from build123d import *

# Parameters (mm, degrees)
F0_W     = 75
F0_H     = 58
F1_DEPTH = 10.5
F3_R     = 5.24999
F4_DEPTH = 6
F5_W     = 6.9
F5_H     = 0.25
F6_DEPTH = 4.572


# Not quite as in the source:
# - a fillet or chamfer is up to 0.001 mm smaller than in the source, because OpenCascade refuses the exact size


with BuildPart() as f1:
    # F0 (on Top) → F1 (new body)
    with BuildSketch(Plane.XY):
        with Locations((-17.9516240954, -13.4977242947)):
            Rectangle(F0_W, F0_H)
    extrude(amount=F1_DEPTH)

    # F3 (radius 5.25 in the source; OpenCascade refuses exactly that, so slightly less here)
    f3_edges = [f1.edges().sort_by_distance(p)[0] for p in [
        (-17.951624, -42.497724, 10.5),
        (-17.951624, -42.497724, 0),
        (-17.951624, 15.502276, 10.5),
        (-17.951624, 15.502276, 0),
    ]]
    fillet(f3_edges, radius=F3_R)

    # F2 (on face) → F4 (cut)
    with BuildSketch(Plane.YZ.offset(19.5483759046)):
        with BuildLine():
            Line((-10.0477242947, 8), (-13.4977242947, 8))
            Line((-13.4977242947, 8), (-16.9477242947, 8))
            ThreePointArc((-16.9477242947, 8), (-15.8517087838, 7.5460155108), (-15.3977242947, 6.45))
            ThreePointArc((-15.3977242947, 6.45), (-15.8517087838, 5.3539844892), (-16.9477242947, 4.9))
            Line((-16.9477242947, 4.9), (-10.0477242947, 4.9))
            ThreePointArc((-10.0477242947, 4.9), (-11.5977242947, 6.45), (-10.0477242947, 8))
        make_face()
        with BuildLine():
            Line((-10.0477242947, 4.9), (-10.0477242947, 8))
            ThreePointArc((-10.0477242947, 8), (-11.5977242947, 6.45), (-10.0477242947, 4.9))
        make_face()
        with BuildLine():
            ThreePointArc((-8.4977242947, 6.45), (-8.9517087838, 7.5460155108), (-10.0477242947, 8))
            Line((-10.0477242947, 8), (-10.0477242947, 4.9))
            ThreePointArc((-10.0477242947, 4.9), (-8.9517087838, 5.3539844892), (-8.4977242947, 6.45))
        make_face()
        with BuildLine():
            ThreePointArc((-15.3977242947, 6.45), (-15.8517087838, 7.5460155108), (-16.9477242947, 8))
            Line((-16.9477242947, 8), (-16.9477242947, 4.9))
            ThreePointArc((-16.9477242947, 4.9), (-15.8517087838, 5.3539844892), (-15.3977242947, 6.45))
        make_face()
        with BuildLine():
            Line((-16.9477242947, 4.9), (-16.9477242947, 8))
            ThreePointArc((-16.9477242947, 8), (-18.0437398055, 7.5460155108), (-18.4977242947, 6.45))
            ThreePointArc((-18.4977242947, 6.45), (-18.0437398055, 5.3539844892), (-16.9477242947, 4.9))
        make_face()
    extrude(amount=-F4_DEPTH, mode=Mode.SUBTRACT)

    # F5 (on face) → F6 (join)
    with BuildSketch(Plane.YZ.offset(13.5483759046)):
        with Locations((-13.4977242947, 6.575)):
            Rectangle(F5_W, F5_H)
        with Locations((-13.4977242947, 6.325)):
            Rectangle(F5_W, F5_H)
    extrude(amount=F6_DEPTH)


solid = f1.part
Check sheet for the modelled part. Datum: model origin and axes. Units: mm. A direction names the side the tool comes from. Round coordinates to 2 decimals unless told otherwise and drop trailing zeros. Loops run counter-clockwise (first coordinate to the right, second up) from the corner with the lowest first, then second, coordinate; pieces in that order, holes last. Notation, with made-up numbers: (35.5, 37.5) -> (58.5, 37.5) arc R34 cw to (58.5, 68.5) -> close; hole circle Ø6 at (25.5, 5). An arc over 180 degrees is marked (long way). Put each result on its own line as item: value. Start each with the question number.
1. Gauge pin test, flat ends, axial feed: pin 1 (5 mm diameter, centred on x = -46.5, z = 1.5, fed in from -Y); pin 2 (0.6 mm diameter, centred on y = -13.5, z = 6.5, fed in from +X); pin 3 (3 mm diameter, centred on x = -17, z = 3.5, fed in from -Y). Record the tip position at first contact, or that the pin passes through.
2. Section check C-C (z = 1.25). Enter the section's corners in (x, y).
3. Draft check along Z on faces 3 (the face through (-17.427, 14.005, 8.921)), 4 (the face through (13.548, -14, 6)), 5 (the face through (-18, -13, 0)). Enter one of: +Z half, -Z half, draft (parallel to the pull), parting line (faces both ways), or undercut.
4. Scan lines: probe 1 along X at (y, z) = (-17.5, 5.5); probe 2 along Z at (x, y) = (-26, -37.5); probe 3 along Y at (x, z) = (-1, 3.25). Record each from-to range of solid material in increasing order.
5. Access from +Z, -Z, +X, -X, +Y, -Y to the whole of each face (thin tool, end or side, straight path). Record for faces 1 (the face through (17, -14, 4.9)), 2 (the face through (-17.43, -41, 8.92)).
6. Section check B-B (y = -13.5). Enter the section's corners in (x, z), plus the area to 3 significant figures.
Findings:
1. pin 1: stops at y = -42.35
1. pin 2: stops at x = 18.12
1. pin 3: stops at y = -42.49
2. outline: (-55.45, -40.65) -> (19.55, -40.65) -> (19.55, 13.65) -> (-55.45, 13.65) -> close
3. face 3: +Z half
3. face 4: undercut
3. face 5: -Z half
4. probe 1: x = -55.45 to 13.55
4. probe 2: z = 0.01 to 10.49
4. probe 3: y = -42.1 to 15.11
5. face 1: +X
5. face 2: +Z, +X, -X, -Y
6. outline: (-55.45, 0) -> (19.55, 0) -> (19.55, 4.9) -> (13.55, 4.9) -> (13.55, 6.2) -> (18.12, 6.2) -> (18.12, 6.7) -> (13.55, 6.7) -> (13.55, 8) -> (19.55, 8) -> (19.55, 10.5) -> (-55.45, 10.5) -> close
6. area: 771 mm^2
